Geometry check sheet. Reference: drawing and pictorial views, mm from the part's lowest x, y, z. A direction names the side the tool comes from. Round coordinates to 2 decimals unless told otherwise and drop trailing zeros. Write each loop counter-clockwise with the first axis right and the second up, starting at its lowest first coordinate (ties: lowest second). Pieces come first, ordered by that corner, then holes.
Item 1: Release check for a two-part mould opening along X. For the marked faces 1, 2 and 3 record: pulls with the +X half, pulls with the -X half, needs draft (parallel to the pull), parting line crosses it, or undercut.
Item 2: Set-up check for the marked faces 4 and 5: record each of +Z, -Z, +X, -X, +Y, -Y from which the full face is reachable in a straight line by a thin tool's end or side.
Item 3: Section check B-B, the plane z = 2. Record the cut outline in (x, y), plus the area to 3 significant figures.
Item 4: Material ranges on line 1 along X through (y, z) = (10, 3.5); line 2 along X through (y, z) = (3.5, 5.75); line 3 along X through (y, z) = (10.5, 8.75), recorded low to high.
Item 5: Section check A-A, the plane x = 74.5. Record the cut outline in (y, z).
Item 6: Section check C-C, the plane y = 10. Record the cut outline in (x, z), plus the area to 3 significant figures.
Item 7: Depth check by flat-ended pin: pin 1 (5 mm diameter, centred on x = 53, y = 13.5, fed in from -Z); pin 2 (1.6 mm diameter, centred on x = 74.5, y = 10, fed in from -Z). Enter the tip coordinate at first touch or a pass-through.
Item 8: Section check D-D, the plane x = 34. Record the cut outline in (y, z).
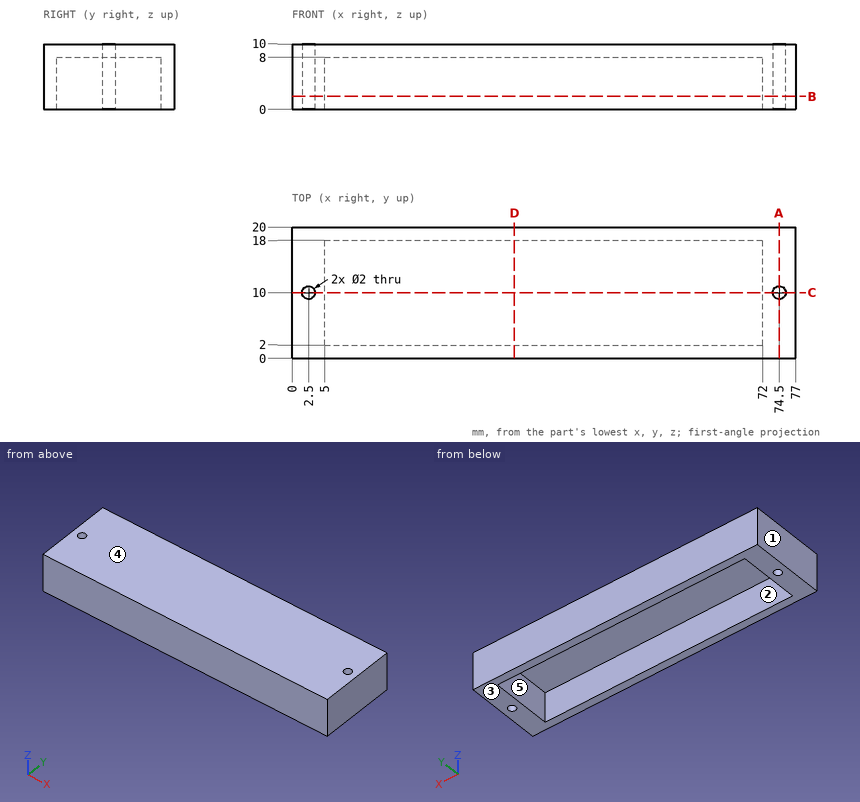
Values found:
1. face 1: pulls with the -X half
1. face 2: undercut
1. face 3: needs draft
2. face 4: +Z, +X, -X, +Y, -Y
2. face 5: -Z
3. outline: (0, 0) - (77, 0) - (77, 20) - (0, 20) - close; hole circle Ø2 at (2.5, 10); hole (5, 2) - (72, 2) - (72, 18) - (5, 18) - close; hole circle Ø2 at (74.5, 10)
3. area: 462 mm2
4. line 1: x = 0 to 1.5, 3.5 to 5, 72 to 73.5, 75.5 to 77
4. line 2: x = 0 to 5, 72 to 77
4. line 3: x = 0 to 1.63, 3.37 to 73.63, 75.37 to 77
5. outline: (0, 0) - (9, 0) - (9, 10) - (0, 10) - close; (11, 0) - (20, 0) - (20, 10) - (11, 10) - close
6. outline: (0, 0) - (1.5, 0) - (1.5, 10) - (0, 10) - close; (3.5, 0) - (5, 0) - (5, 8) - (72, 8) - (72, 0) - (73.5, 0) - (73.5, 10) - (3.5, 10) - close; (75.5, 0) - (77, 0) - (77, 10) - (75.5, 10) - close
6. area: 194 mm2
7. pin 1: stops at z = 8
7. pin 2: passes through
8. outline: (0, 0) - (2, 0) - (2, 8) - (18, 8) - (18, 0) - (20, 0) - (20, 10) - (0, 10) - close
